Autodesk Inventor part; units mm, degrees
ref_plane "YZ Plane" through (0, 0, 0) normal (1, 0, 0) x (0, 1, 0)
ref_plane "XZ Plane" through (0, 0, 0) normal (0, 1, 0) x (-1, 0, 0)
ref_plane "XY Plane" through (0, 0, 0) normal (0, 0, 1) x (1, 0, 0)
sketch "Náčrt1" plane through (0, 0, 0) normal (0, 0, 1) x (1, 0, 0)
  line L0 (0, 7) -> (0, -7)
  line L1 (-7, 0) -> (7, 0)
  line L2 (-3.5, 3.5) -> (3.5, 3.5)
  line L3 (3.5, 3.5) -> (3.5, -3.5)
  line L4 (3.5, -3.5) -> (-3.5, -3.5)
  line L5 (-3.5, -3.5) -> (-3.5, 3.5)
  line L6 (-5, 5) -> (5, 5)
  line L7 (5, 5) -> (5, -5)
  line L8 (5, -5) -> (-5, -5)
  line L9 (-5, -5) -> (-5, 5)
  point P0 (0, 0)
  dimension "d1" = 10
  dimension "d2" = 10
  dimension "d3" = 1.5
  dimension "d4" = 1.5
  dimension "d5" = 1.5
  dimension "d6" = 1.5
extrude "Vysunutí1" add sketch "Náčrt1" along normal mid plane 22.5 contours L6 L7 L1 L3 L2 L0 | L0 L2 L5 L1 L9 L6 | L1 L5 L4 L0 L8 L9 | L7 L8 L0 L4 L3 L1
sketch "Náčrt2" plane through (-5, 5, 11.25) normal (0, 1, 0) x (1, 0, 0)
  line L0 (12, 11.25) -> (-2, 11.25)
  line L1 (5, 27) -> (5, -4.5)
  line L2 (10, 0) -> (0, 0)
  line L3 (0, 22.5) -> (0, 0)
  point P0 (5, 11.25)
  point P1 (5, 5)
  dimension "d10" = 5
  dimension "d11" = 5
hole "Díra1" at (0, 5, 6.25) direction (0, -1, 0) diameter 3.2 end through all counterbore diameter 6.5 counterbore depth 2
sketch "Náčrt3" plane through (-5, 5, 11.25) normal (0, 1, 0) x (1, 0, 0)
  line L0 (0, 22.5) -> (0, 0)
  line L1 (0, 22.5) -> (10, 22.5)
  point P0 (5, 11.25)
  point P1 (5, 15)
  point P2 (5, 3)
  dimension "d19" = 5
  dimension "d20" = 5
  dimension "d21" = 12
  dimension "d22" = 7.5
hole "Díra2" at (0, 5, -3.75) at (0, 5, 8.25) direction (0, -1, 0) diameter 2.459 depth 1.5
mirror "Zrcadlit1" about plane through (0, 0, -11.25) normal (0, 0, -1) of "Vysunutí1", "Díra1", "Díra2"
properties part number "bearing_base" material "Hliník 6061"
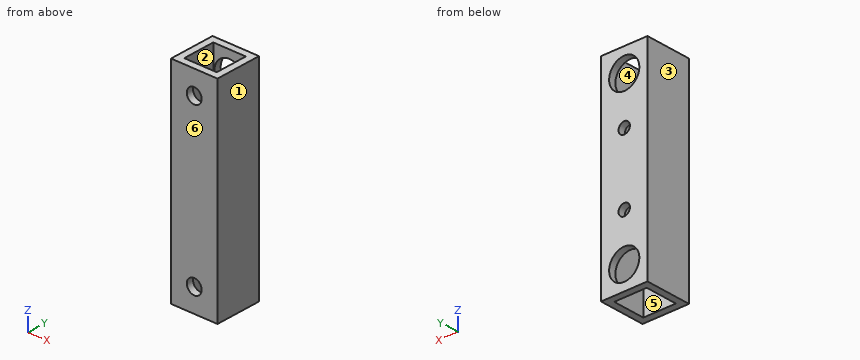
Input: part model. Units: mm. Frame: model coordinates. Face numbers are marked on the shaded views. A direction names the side the tool comes from. Give positions to 0.01 mm unless a question says otherwise; leave off trailing zeros. Order: outer loops, then holes, each group sorted by start corner. A loop starts at its lowest first (then second) coordinate and runs counter-clockwise, first axis right, second up. Notation, with made-up numbers: M -17,-20.75 L 14,-20.75 A33 ccw 14,9.25 Z; hole C 65,69.25 d5. An arc over 180 degrees is marked long. One line per question, with ' | ' between items. Start each with the question number.
1. Section query D-D (x = 2). Return the cut outline in (y, z), and give its area (3 significant figures).
2. First-contact query: pin 1 Ø4 at (x, z) = (0, 6.25) entering from +Y; pin 2 Ø3 at (x, z) = (0, -28.75) entering from +Y; pin 3 Ø3.5 at (x, z) = (0, 6.25) entering from -Y. Flat tips, straight axial feed; report the tip coordinate or a pass-through.
3. Section query C-C (z = -3.75). Return the cut outline in (x, y), and give its area (3 significant figures).
4. Section query B-B (z = -28.75). Return the cut outline in (x, y).
5. Material intervals for probe 1 along Z at (x, y) = (0, 4.6); probe 2 along X at (y, z) = (4.55, -28.75); probe 3 along Y at (x, z) = (-2, -25.5), sorted ascending. Write a range as [from, to].
6. Section query A-A (y = -0.5). Return the cut outline in (x, z).
7. Access query for the marked faces 1 and 2. Directions: +Z, -Z, +X, -X, +Y, -Y. A direction counts if a zero-diameter tool reaches every point of the face in a straight line with its end or side. Return the directions, or none.
8. Pull-direction query (Y, two-part tool) for the marked faces 3, 4, 5 and 6; classes: released by +Y, released by -Y, zero draft, split by the parting line, or undercut.
Here are the results:
1) outline: M -5,-33.75 L -3.5,-33.75 L -3.5,11.25 L -5,11.25 Z; M 3.5,-33.75 L 5,-33.75 L 5,-31.31 L 3.5,-31.31 Z; M 3.5,-26.19 L 5,-26.19 L 5,3.69 L 3.5,3.69 Z; M 3.5,8.81 L 5,8.81 L 5,11.25 L 3.5,11.25 Z | area: 120 mm²
2) pin 1: y = -3.5 | pin 2: through | pin 3: y = -5
3) outline: M -5,-5 L 5,-5 L 5,5 L 1.23,5 L 1.23,3.5 L 3.5,3.5 L 3.5,-3.5 L -3.5,-3.5 L -3.5,3.5 L -1.23,3.5 L -1.23,5 L -5,5 Z | area: 47.3 mm²
4) outline: M -5,-5 L -1.6,-5 L -1.6,-3.5 L -3.5,-3.5 L -3.5,3.5 L -3.25,3.5 L -3.25,5 L -5,5 Z; M 1.6,-5 L 5,-5 L 5,5 L 3.25,5 L 3.25,3.5 L 3.5,3.5 L 3.5,-3.5 L 1.6,-3.5 Z
5) probe 1: [-33.75, -32], [-25.5, -19.98], [-17.52, -4.98], [-2.52, 3], [9.5, 11.25] | probe 2: [-5, -3.25], [3.25, 5] | probe 3: [-5, -3.5], [3.5, 5]
6) outline: M -5,-33.75 L -3.5,-33.75 L -3.5,11.25 L -5,11.25 Z; M 3.5,-33.75 L 5,-33.75 L 5,11.25 L 3.5,11.25 Z
7) face 1: +Z, -Z, +X, +Y, -Y | face 2: +Z, -Z
8) face 3: zero draft | face 4: undercut | face 5: undercut | face 6: released by -Y
